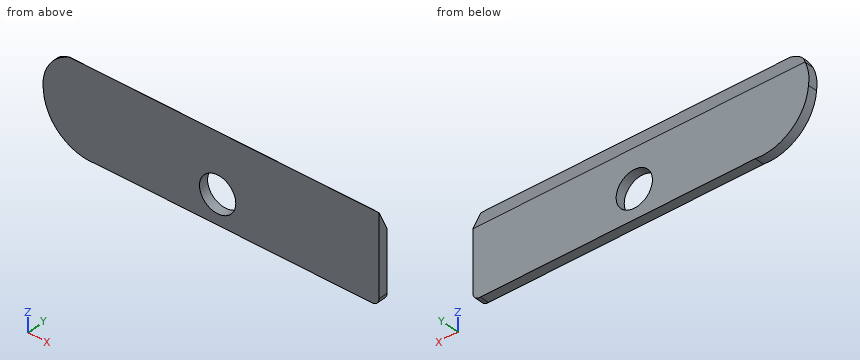
from build123d import *

# Parameters (mm, degrees)
F0_R     = 1.35
F1_DEPTH = 0.7
F2_R     = 1.35
F3_DEPTH = 25
F5_DEPTH = 25


with BuildPart() as f1:
    # F0 (on Front) → F1 (new body)
    with BuildSketch(Plane.XZ):
        with BuildLine():
            Line((-21, 0), (-0.5443152335, -0.0158934575))
            ThreePointArc((-0.5443152335, -0.0158934575), (-0.1558427945, 0.1191114487), (0, 0.499703335))
            Line((0, 0.499703335), (0, 4.9841065425))
            Line((0, 4.9841065425), (-24.6915577171, 4.9841065425))
            ThreePointArc((-24.6915577171, 4.9841065425), (-24.951684375, 4.1365627533), (-24.95, 3.25))
            ThreePointArc((-24.95, 3.25), (-23.6789862708, 0.769385917), (-21, 0))
        make_face()
        with Locations((-12.475, 2.15)):
            Circle(F0_R, mode=Mode.SUBTRACT)
        with BuildLine():
            Line((-24.6915577171, 4.9841065425), (0, 4.9841065425))
            Line((0, 4.9841065425), (0, 6.5))
            Line((0, 6.5), (-23, 6.5))
            ThreePointArc((-23, 6.5), (-23.9964550111, 5.9101900274), (-24.6915577171, 4.9841065425))
        make_face()
        with Locations((-12.475, 2.15)):
            Circle(F0_R)
    extrude(amount=F1_DEPTH)

    # F2 (on face) → F3 (cut)
    with BuildSketch(Plane.XZ.offset(0.7)):
        with Locations((-11.9948536158, 2.1341065425)):
            Circle(F2_R)
    extrude(amount=-F3_DEPTH, mode=Mode.SUBTRACT)

    # F4 (on Right) → F5 (cut)
    with BuildSketch(Plane.YZ):
        Polygon((-0.7018046454, 6.5234168433), (0, 5), (0, 6.521099247), align=None)
    extrude(amount=-F5_DEPTH, mode=Mode.SUBTRACT)


solid = f1.part
The listing builds one solid part. Answer for the finished solid, in the listing's coordinates (mm). Give positions to 0.01 mm unless a question says otherwise; leave off trailing zeros. Write each loop counter-clockwise with the first axis right and the second up, starting at its lowest first coordinate (ties: lowest second). Pieces come first, ordered by that corner, then holes. Notation, with made-up numbers: (28, -0.5) - (40, -0.5) arc R34 cw to (40, 33.5) - close; hole circle Ø5 at (49, 75.5). An arc over 180 degrees is marked (long way). One line per question, with ' | ' between items. Start each with the question number.
1. Section B-B, the plane z = 3 is taken. Determine the outline of the cut face in (x, y).
2. Straight lines are drawn through the part: line 1 (X direction, y = -0.4, z = 1.75); line 2 (X direction, y = -0.2, z = 1.25); line 3 (Z direction, x = -12, y = -0.55). For each, find the intervals that lie inside material, in ascending order.
3. Section A-A, the plane y = -0.55 is taken. Determine the outline of the cut face in (x, z).
Result:
1) outline: (-24.92, -0.7) - (-13.03, -0.7) - (-13.03, 0) - (-24.92, 0) - close; (-10.96, -0.7) - (0, -0.7) - (0, 0) - (-10.96, 0) - close
2) line 1: x = -24.5 to -13.29, -10.7 to 0 | line 2: x = -24.16 to -13.02, -10.97 to 0 | line 3: z = -0.01 to 0.78, 3.48 to 6.19
3) outline: (-24.95, 3.25) arc R3.51 ccw to (-21, 0) - (-0.54, -0.02) arc R0.5 ccw to (0, 0.5) - (0, 6.19) - (-23.62, 6.19) arc R2.97 ccw to start; hole circle Ø2.7 at (-11.99, 2.13)
